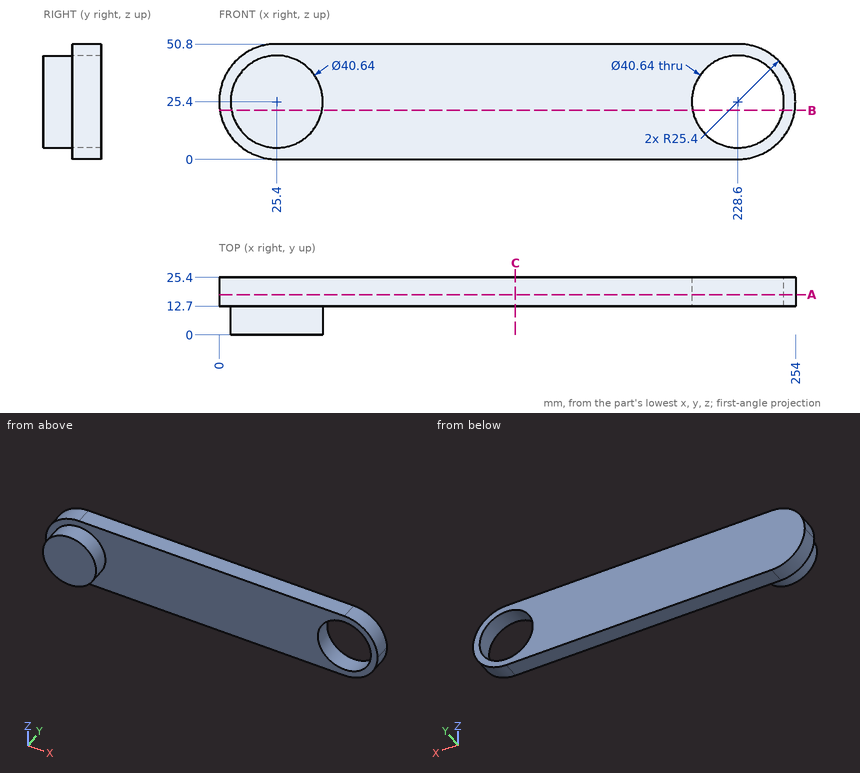
Source: three-view drawing plus pictorial views. Frame: mm from the lowest corner of the part. Round coordinates to 2 decimals unless told otherwise and drop trailing zeros. Order: outer loops, then holes, each group sorted by start corner. A loop starts at its lowest first (then second) coordinate and runs counter-clockwise, first axis right, second up. Notation, with made-up numbers: (11.25, -7.75) -> (15.25, -7.75) arc R17 ccw to (15.25, 9.25) -> close; hole circle Ø7 at (48.5, 23). An arc over 180 degrees is marked (long way). Use one line per item in the form item = value. Start each with the question number.
1. Cut plane B-B (z = 21.5). Return the cut outline in (x, y).
2. Cut plane C-C (x = 130.5). Return the cut outline in (y, z), then the cut area to 3 significant figures.
3. Line query: probe 1 along Y at (x, z) = (142, 4); probe 2 along Z at (x, y) = (214, 23); probe 3 along X at (y, z) = (13.75, 18). Output: solid intervals per line, ascending.
4. Cut plane A-A (y = 17.75). Return the cut outline in (x, z).
5. Pin query (flat end, axial travel): pin 1 Ø12 at (y, z) = (16, 38) entering from -X; pin 2 Ø8 at (y, z) = (22.5, 8.5) entering from -X; pin 3 Ø2 at (y, z) = (13.5, 29) entering from -X. Return the tip coordinate at first contact, or that it passes through.
Solution:
q1.outline = (0.3, 12.7) -> (5.46, 12.7) -> (5.46, 0) -> (45.34, 0) -> (45.34, 12.7) -> (208.66, 12.7) -> (208.66, 25.4) -> (0.3, 25.4) -> close; (248.54, 12.7) -> (253.7, 12.7) -> (253.7, 25.4) -> (248.54, 25.4) -> close
q2.outline = (12.7, 0) -> (25.4, 0) -> (25.4, 50.8) -> (12.7, 50.8) -> close
q2.area = 645 mm^2
q3.probe_1 = 12.7 to 25.4
q3.probe_2 = 0 to 11.27, 39.53 to 50.8
q3.probe_3 = 1.1 to 209.68, 247.52 to 252.9
q4.outline = (25.4, 0) -> (228.6, 0) arc R25.4 ccw to (228.6, 50.8) -> (25.4, 50.8) arc R25.4 ccw to start; hole circle Ø40.64 at (228.6, 25.4)
q5.pin_1 = 0.87
q5.pin_2 = 3.52
q5.pin_3 = 0.13
